from build123d import *

# Parameters (mm, degrees)
SKETCH_1_W      = 114.3
SKETCH_1_H      = 28.5
EXTRUDE_1_DEPTH = 10
HOLE_WIZARD_1_D = 3.175


with BuildPart() as part:
    # 스케치1 → 보스-돌출1 (new body)
    with BuildSketch(Plane.XY):
        with Locations((57.15, 14.25)):
            Rectangle(SKETCH_1_W, SKETCH_1_H)
    extrude(amount=EXTRUDE_1_DEPTH)

    # 구멍1 (through all)
    with Locations(Plane.XY.offset(10)):
        with Locations((18.796, 22.98125), (111.665004, 22.98125), (10.16, 14.25)):
            hole_wizard_1 = Hole(HOLE_WIZARD_1_D / 2)

    # 대칭 복사1: 구멍1 across plane
    add(hole_wizard_1.mirror(Plane.ZX.offset(14.25)), mode=Mode.SUBTRACT)


solid = part.part
Geometry check sheet. Reference: the model listing, model coordinates, mm. Give positions to 0.01 mm unless a question says otherwise; leave off trailing zeros. Order: outer loops, then holes, each group sorted by start corner. A loop starts at its lowest first (then second) coordinate and runs counter-clockwise, first axis right, second up.
1) Cross-section at A-A (x = 10.16). Record the boundary of the cut face in (y, z), then the cut area to 3 significant figures.
Results are:
outline: (0, 0) - (12.66, 0) - (12.66, 10) - (0, 10) - close; (15.84, 0) - (28.5, 0) - (28.5, 10) - (15.84, 10) - close
area: 253 mm2
2) Gauge pin test, flat end, axial feed: pin 1 (2.5 mm diameter, centred on x = 18.8, y = 22.98, fed in from -Z). Record the tip position at first contact, or that the pin passes through.
Results are:
pin 1: passes through
3) Draft check along X on faces 1 (the cylindrical face through (113.25, 23.05, 4.93)), 2 (the flat face through (56, 14, 10)), 3 (the cylindrical face through (19.97, 4.45, 4.93)), 4 (the flat face through (114.3, 14, 5)). Enter one of: released by +X, released by -X, zero draft, split by the parting line, or undercut.
Results are:
face 1: undercut
face 2: zero draft
face 3: undercut
face 4: released by +X
4) Material ranges on probe 1 along X at (y, z) = (23.25, 6.5); probe 2 along X at (y, z) = (5.5, 7.25); probe 3 along Y at (x, z) = (10.16, 3.25), recorded low to high.
Results are:
probe 1: x = 0 to 17.23, 20.36 to 110.1, 113.23 to 114.3
probe 2: x = 0 to 17.21, 20.38 to 110.08, 113.25 to 114.3
probe 3: y = 0 to 12.66, 15.84 to 28.5
5) Cross-section at B-B (y = 14.25). Record the boundary of the cut face in (x, z), then the cut area to 3 significant figures.
Results are:
outline: (0, 0) - (8.57, 0) - (8.57, 10) - (0, 10) - close; (11.75, 0) - (114.3, 0) - (114.3, 10) - (11.75, 10) - close
area: 1,110 mm2
